from build123d import *

# Parameters (mm, degrees)
CROQUIS1_R              = 10
SALIENTE_EXTRUIR2_DEPTH = 8


with BuildPart() as part:
    # Croquis1 → Saliente-Extruir2 (new body)
    with BuildSketch(Plane.XY):
        with BuildLine():
            ThreePointArc((-62.5, 12.951833847), (0, 38.192664612), (62.5, 12.951833847))
            ThreePointArc((62.5, 12.951833847), (63.839595947, -11.509369402), (39.544117647, -14.651775463))
            ThreePointArc((39.544117647, -14.651775463), (28.573082694, -11.763695145), (18.445121951, -16.875351143))
            ThreePointArc((18.445121951, -16.875351143), (0, -25), (-18.445121951, -16.875351143))
            ThreePointArc((-18.445121951, -16.875351143), (-28.573082694, -11.763695145), (-39.544117647, -14.651775463))
            ThreePointArc((-39.544117647, -14.651775463), (-63.839595947, -11.509369402), (-62.5, 12.951833847))
        make_face()
        with Locations((-50, 0)):
            Circle(CROQUIS1_R, mode=Mode.SUBTRACT)
        with Locations(Location((50, 0, 0), (0, 0, 180))):
            Circle(CROQUIS1_R, mode=Mode.SUBTRACT)
        with BuildLine():
            Line((4, 14.456832295), (4, 23))
            Line((4, 23), (-4, 23))
            Line((-4, 23), (-4, 14.456832295))
            ThreePointArc((-4, 14.456832295), (0, -15), (4, 14.456832295))
        make_face(mode=Mode.SUBTRACT)
    extrude(amount=SALIENTE_EXTRUIR2_DEPTH)


solid = part.part
Verification items for the finished model (mm, model axes). A direction names the side the tool comes from. Give positions to 0.01 mm unless a question says otherwise; leave off trailing zeros. Order: outer loops, then holes, each group sorted by start corner. A loop starts at its lowest first (then second) coordinate and runs counter-clockwise, first axis right, second up. Notation, with made-up numbers: M 51,-31 L 91,-31 A15 cw 91,-14 Z; hole C 88,80.5 d7. An arc over 180 degrees is marked long. Use one line per item in the form item = value. Start each with the question number.
Q1. Mould release check, pull along X, two halves, no side actions. Record for faces 3 (the flat face through (-14, 7, 8)), 4 (the cylindrical face through (-0.967, 38.187, 3.944)), 5 (the cylindrical face through (64.078, -11.217, 3.944)): +X half, -X half, draft (parallel to the pull), parting line (faces both ways), or undercut.
Q2. Section check A-A (y = 0). Enter the section's corners in (x, z), then the cut area to 3 significant figures.
Q3. Section check D-D (y = 19.5). Enter the section's corners in (x, z).
Q4. Go/stop test with flat-tipped pins: pin 1 Ø10 at (x, y) = (19.5, 12.5) entering from -Z; pin 2 Ø3 at (x, z) = (21, 7) entering from -Y; pin 3 Ø3 at (y, z) = (-7, 1.5) entering from -X; pin 4 Ø2 at (x, z) = (24, 1) entering from -Y. Record where each tip stops, or that it passes through.
Q5. Section check C-C (z = 6.75). Enter the section's corners in (x, y), then the cut area to 3 significant figures.
Q6. Section check B-B (x = 0). Enter the section's corners in (y, z), then the cut area to 3 significant figures.
Q7. Scan lines: line 1 along X through (y, z) = (-8, 1.5); line 2 along Y through (x, z) = (50, 5.5); line 3 along X through (y, z) = (2, 6.5). Record each from-to range of solid material in increasing order. Write a range as [from, to].
Q8. Access from +Z, -Z, +X, -X, +Y, -Y to the whole of each face (thin tool, end or side, straight path). Record for faces 1 (the flat face through (4, 19, 4)), 2 (the cylindrical face through (-28.41, -11.78, 3.94)).
Evaluation:
q1.face_3 = draft
q1.face_4 = parting line
q1.face_5 = undercut
q2.outline = M -68,0 L -60,0 L -60,8 L -68,8 Z; M -40,0 L -15,0 L -15,8 L -40,8 Z; M 15,0 L 40,0 L 40,8 L 15,8 Z; M 60,0 L 68,0 L 68,8 L 60,8 Z
q2.area = 528 mm2
q3.outline = M -54.91,0 L -4,0 L -4,8 L -54.91,8 Z; M 4,0 L 54.91,0 L 54.91,8 L 4,8 Z
q4.pin_1 = 0
q4.pin_2 = -15.82
q4.pin_3 = -67.14
q4.pin_4 = -13.41
q5.outline = M -62.5,12.95 A18 ccw -39.54,-14.65 A16 cw -18.45,-16.88 A25 ccw 18.45,-16.88 A16 cw 39.54,-14.65 A18 ccw 62.5,12.95 A90 ccw Z; hole C -50,0 d20; hole M -4,14.46 A15 ccw long 4,14.46 L 4,23 L -4,23 Z; hole C 50,0 d20
q5.area = 4,730 mm2
q6.outline = M -25,0 L -15,0 L -15,8 L -25,8 Z; M 23,0 L 38.19,0 L 38.19,8 L 23,8 Z
q6.area = 202 mm2
q7.line_1 = [-66.12, -56], [-44, -12.69], [12.69, 44], [56, 66.12]
q7.line_2 = [-18, -10], [10, 23.03]
q7.line_3 = [-67.89, -59.8], [-40.2, -14.87], [14.87, 40.2], [59.8, 67.89]
q8.face_1 = +Z, -Z
q8.face_2 = +Z, -Z, -Y
